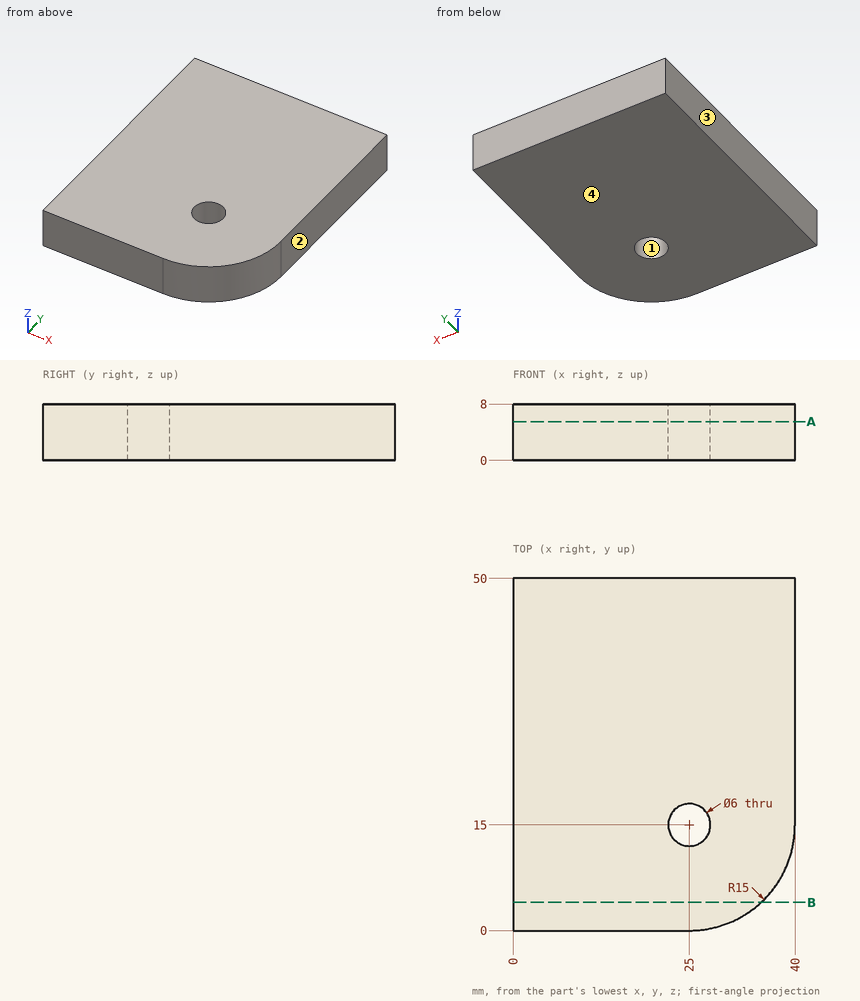
Geometry check sheet. Reference: drawing and pictorial views, mm from the part's lowest x, y, z. Round coordinates to 2 decimals unless told otherwise and drop trailing zeros. Order: outer loops, then holes, each group sorted by start corner. A loop starts at its lowest first (then second) coordinate and runs counter-clockwise, first axis right, second up. Notation, with made-up numbers: (-37.5, 81) - (-4.5, 81) arc R8 ccw to (-4.5, 85) - close; hole circle Ø5 at (-35, -20). An arc over 180 degrees is marked (long way). Use a Markdown table: item, result. Add a question column.
1) Mould release check, pull along X, two halves, no side actions. Record for the marked faces 1, 2, 3 and 4: released by +X, released by -X, zero draft, split by the parting line, or undercut.
2) Section check B-B (y = 4). Record the cut outline in (x, z).
3) Thickness scan on line 1 along X through (y, z) = (15, 4.75); line 2 along Y through (x, z) = (25, 3); line 3 along X through (y, z) = (16.5, 0.75). Record the ranges inside material, lowest first.
4) Section check A-A (z = 5.5). Record the cut outline in (x, y), then the cut area to 3 significant figures.
5) Gauge pin test, flat end, axial feed: P1, Ø3, axis at x = 31, z = 4, coming from the -Y side. Record the tip position at first contact, or that the pin passes through.
Established:
| question | item | result |
|---|---|---|
| 1 | face 1 | undercut |
| 1 | face 2 | released by +X |
| 1 | face 3 | released by -X |
| 1 | face 4 | zero draft |
| 2 | outline | (0, 0) - (35.2, 0) - (35.2, 8) - (0, 8) - close |
| 3 | line 1 | 0 to 22, 28 to 40 |
| 3 | line 2 | 0 to 12, 18 to 50 |
| 3 | line 3 | 0 to 22.4, 27.6 to 40 |
| 4 | outline | (0, 0) - (25, 0) arc R15 ccw to (40, 15) - (40, 50) - (0, 50) - close; hole circle Ø6 at (25, 15) |
| 4 | area | 1,920 mm2 |
| 5 | P1 | y = 0.69 |
